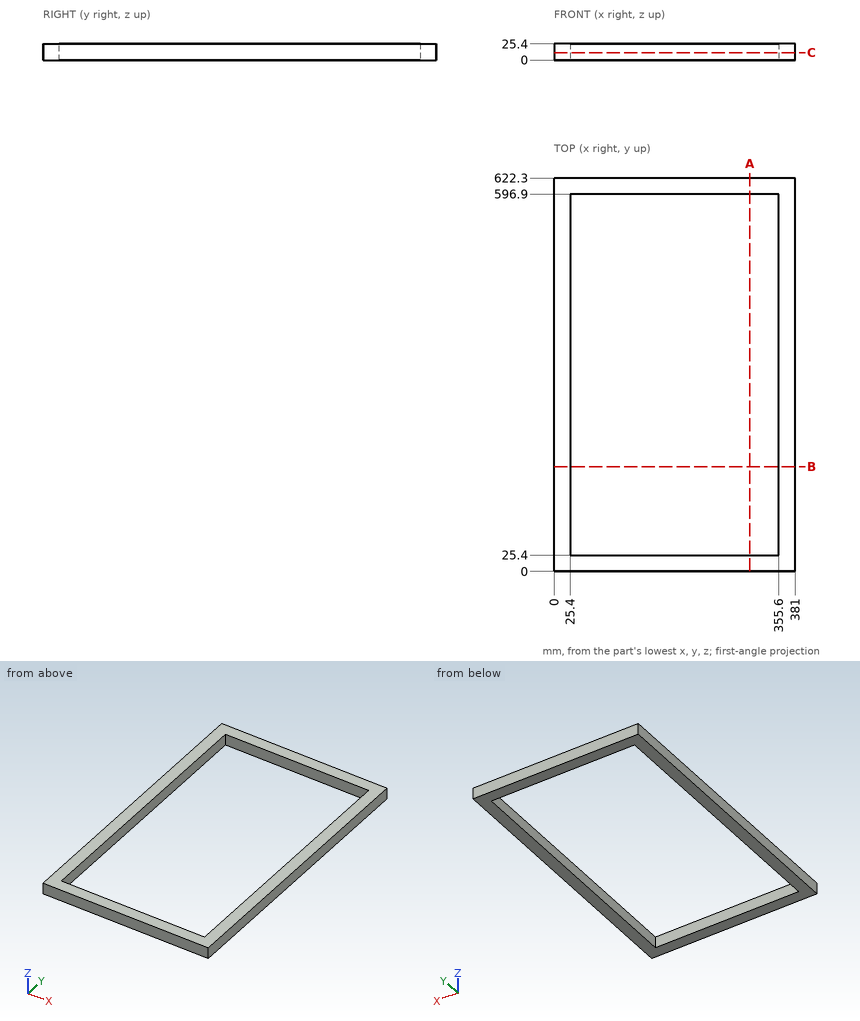
Drawing for the job (mm, zero at the part's lowest x, y, z). Coordinates: 2 decimals unless noted, no trailing zeros. Loops run counter-clockwise (first coordinate to the right, second up) from the corner with the lowest first, then second, coordinate; pieces in that order, holes last. Notation, with made-up numbers: (10.5, 63) - (54.5, 63) arc R32 cw to (54.5, 98) - close; hole circle Ø3 at (10.25, 45.5). An arc over 180 degrees is marked (long way). Return JSON: item names as keys, results as strings.
1. Probe L1, parallel to X at y = 497, z = 6.5; L2, parallel to Y at x = 230, z = 14.25. List the from-to ranges inside material, lowest first. Write a range as from..to.
Result:
{"L1": "x = 0..25.4, 355.6..381", "L2": "y = 0..25.4, 596.9..622.3"}
2. Band-saw the part on A-A (x = 309.5). Give the cut face in (y, z), and give its area (3 significant figures).
Result:
{"outline": "(0, 0) - (25.4, 0) - (25.4, 25.4) - (0, 25.4) - close; (596.9, 0) - (622.3, 0) - (622.3, 25.4) - (596.9, 25.4) - close", "area": "1,290 mm2"}
3. Band-saw the part on B-B (y = 165.5). Give the cut face in (x, z).
Result:
{"outline": "(0, 0) - (25.4, 0) - (25.4, 25.4) - (0, 25.4) - close; (355.6, 0) - (381, 0) - (381, 25.4) - (355.6, 25.4) - close"}
4. Band-saw the part on C-C (z = 11.75). Give the cut face in (x, y), and give its area (3 significant figures).
Result:
{"outline": "(0, 0) - (381, 0) - (381, 622.3) - (0, 622.3) - close; hole (25.4, 25.4) - (355.6, 25.4) - (355.6, 596.9) - (25.4, 596.9) - close", "area": "48,400 mm2"}
